The listing builds one solid part. Answer for the finished solid, in the listing's coordinates (mm). Face numbers are marked on the shaded views. A direction names the side the tool comes from. Give positions to 0.01 mm unless a question says otherwise; leave off trailing zeros. Loops run counter-clockwise (first coordinate to the right, second up) from the corner with the lowest first, then second, coordinate; pieces in that order, holes last. Notation, with made-up numbers: M -2,82 L 52,82 A15 ccw 52,100 Z; hole C 34,54.25 d8. An arc over 180 degrees is marked long. Use one line per item in the form item = value. Start each with the question number.
1. Straight lines are drawn through the part: line 1 (X direction, y = -11.5, z = -54); line 2 (X direction, y = -9.5, z = 51); line 3 (Z direction, x = -11, y = -8). For each, find the intervals that lie inside material, in ascending order. Write a range as from..to.
2. For the marked faces 1 and 2, determine the directions among +Z, -Z, +X, -X, +Y, -Y from which every point of the face is accessible in a straight line to the end or side of a thin tool.
3. The part is cut by section B-B (z = -35.5). Write down the section's boundary in (x, y), and give its area (3 significant figures).
4. The part is cut by section A-A (y = -42). Write down the section's boundary in (x, z), and give its area (3 significant figures).
5. Each of these flat-tipped pins is pushed along its axis until it touches: pin 1 Ø10 at (y, z) = (-22.5, 9) entering from -X; pin 2 Ø4 at (x, y) = (5, -10.5) entering from -Z; pin 3 Ø5.5 at (x, y) = (64, -27) entering from -Z. Where does it stop, or does it pass through?
6. The part is cut by section C-C (x = 54). Write down the section's boundary in (y, z).
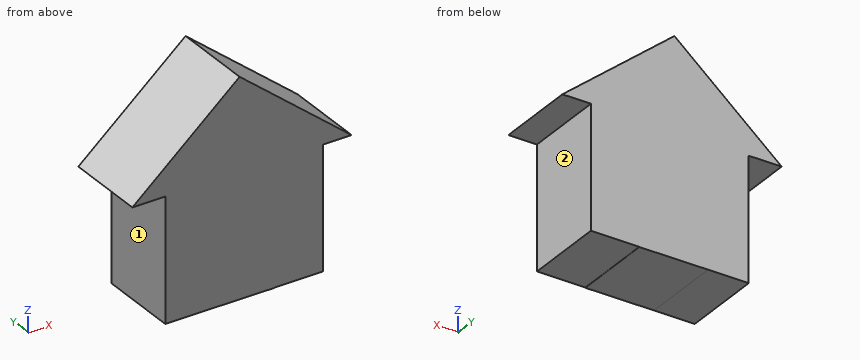
from build123d import *

# Parameters (mm, degrees)
F1_DEPTH = 50.8


with BuildPart() as f1:
    # F0 (on Front) → F1 (new body)
    with BuildSketch(Plane.XZ):
        Polygon((-66.646784544, 0), (-46.1711846292, 0), (51.8861822784, 0), (69.6556717157, 0), (0, 56.993290782), align=None)
        Polygon((51.8861822784, 0), (-46.1711846292, 0), (-46.1711846292, -76.2501358986), (-20.9102912922, -76.1726471121), (-20.9102912922, -21.5385891497), (21.8144096434, -21.5385891497), (21.8144096434, -76.0415874072), (51.8861822784, -75.9493410587), align=None)
        Polygon((-20.9102912922, -21.5385891497), (-20.9102912922, -76.1726471121), (21.8144096434, -76.0415874072), (21.8144096434, -21.5385891497), align=None)
        Polygon((21.8144096434, -76.0415874072), (-20.9102912922, -76.1726471121), (21.8144096434, -76.1726471121), align=None)
    extrude(amount=F1_DEPTH)


solid = f1.part
Derived:
q1.line_1 = -46.17..51.89
q1.line_2 = -7.01..7.32
q1.line_3 = -76.17..47.59
q2.face_1 = -Z, -X, +Y, -Y
q2.face_2 = -Z, +X, +Y, -Y
q3.outline = M -46.17,-50.8 L 51.89,-50.8 L 51.89,0 L -46.17,0 Z
q3.area = 4,980 mm2
q4.outline = M -66.65,0 L -46.17,0 L -46.17,-76.25 L -20.91,-76.17 L 21.81,-76.17 L 21.81,-76.04 L 51.89,-75.95 L 51.89,0 L 69.66,0 L 0,56.99 Z
q4.area = 11,300 mm2
q5.pin_1 = -61.97
q5.pin_2 = -76.17
q5.pin_3 = 0
q6.outline = M -50.8,0 L 0,0 L 0,12.81 L -50.8,12.81 Z
